Could you check a few things on this model? Use its own coordinates, in mm. Give positions to 0.01 mm unless a question says otherwise; leave off trailing zeros. Order: outer loops, then holes, each group sorted by start corner. A loop starts at its lowest first (then second) coordinate and runs counter-clockwise, first axis right, second up. Notation, with made-up numbers: (55, 56) -> (89, 56) arc R23 cw to (89, 84) -> close; hole circle Ø5 at (89.5, 80.5). An arc over 180 degrees is marked (long way). One line per item, written item: value.
```python
from build123d import *

# Parameters (mm, degrees)
F0_W     = 70
F0_H     = 30
F1_DEPTH = 10.8


with BuildPart() as f1:
    # F0 (on Top) → F1 (new body)
    with BuildSketch(Plane.XY):
        with Locations((0, -35.666667)):
            Rectangle(F0_W, F0_H)
        Polygon((-20, 39.333333), (-35, 9.333333), (35, 9.333333), (20, 39.333333), align=None)
        with Locations((0, -5.666667)):
            Rectangle(F0_W, F0_H)
        Polygon((0, 57.333333), (-20, 39.333333), (20, 39.333333), align=None)
    extrude(amount=F1_DEPTH)


solid = f1.part
```
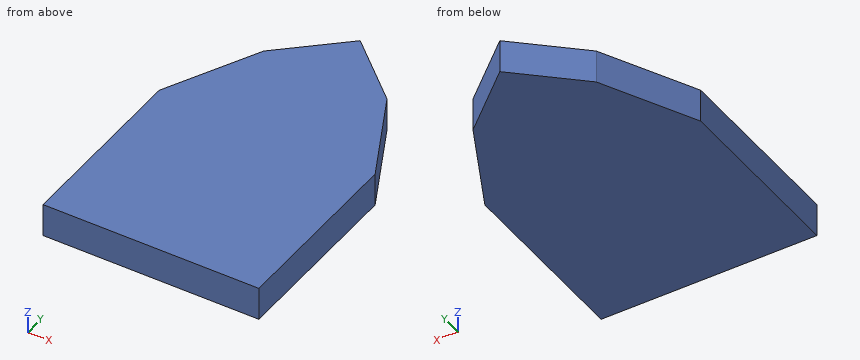
1) Suppose I cut it at C-C, the plane x = -18. Write out the boundary of the cut face in (y, z).
Answer below:
outline: (-50.67, 0) -> (41.13, 0) -> (41.13, 10.8) -> (-50.67, 10.8) -> close
2) Suppose I cut it at B-B, the plane y = 43. Write out the boundary of the cut face in (x, z), then the cut area to 3 significant figures.
Answer below:
outline: (-15.93, 0) -> (15.93, 0) -> (15.93, 10.8) -> (-15.93, 10.8) -> close
area: 344 mm2
3) If I drill on line 1 along X through (y, z) = (28, 2.25); line 2 along Y through (x, z) = (-10, 5.25); line 3 along Y through (x, z) = (-17.5, 8.25), over which ranges is the centre line in solid material (lowest first)?
Answer below:
line 1: x = -25.67 to 25.67
line 2: y = -50.67 to 48.33
line 3: y = -50.67 to 41.58
4) Suppose I cut it at A-A, the plane z = 8. Write out the boundary of the cut face in (x, y), then the cut area to 3 significant figures.
Answer below:
outline: (-35, -50.67) -> (35, -50.67) -> (35, 9.33) -> (20, 39.33) -> (0, 57.33) -> (-20, 39.33) -> (-35, 9.33) -> close
area: 6,210 mm2
5) For P1, Ø3, axis at y = 21.5, z = 1.5, coming from the +X side; P2, Ø6, axis at x = -24, z = 3, coming from the +Y side; P3, Ø1.5, axis at y = 42, z = 2, coming from the -X side, each with a flat end and sliding along its axis, tell me the tip position at first contact or that it passes through.
Answer below:
P1: stops at x = 29.67
P2: stops at y = 37.33
P3: stops at x = -17.87
